from build123d import *

# Parameters (mm, degrees)
SKETCH1_W           = 200
SKETCH1_H           = 200
BOSS_EXTRUDE1_DEPTH = 30
SKETCH3_R           = 75
BOSS_EXTRUDE2_DEPTH = 30
SKETCH4_R           = 15
CUT_EXTRUDE1_DEPTH  = 30


with BuildPart() as part:
    # Sketch1 → Boss-Extrude1 (new body)
    with BuildSketch(Plane(origin=(0, 0, 0), x_dir=(1, 0, 0), z_dir=(0, 1, 0))):
        Rectangle(SKETCH1_W, SKETCH1_H)
    extrude(amount=BOSS_EXTRUDE1_DEPTH)

    # Sketch3 → Boss-Extrude2 (add)
    with BuildSketch(Plane(origin=(0, 30, 0), x_dir=(1, 0, 0), z_dir=(0, 1, 0))):
        Circle(SKETCH3_R)
    extrude(amount=BOSS_EXTRUDE2_DEPTH)

    # Sketch4 → Cut-Extrude1 (cut)
    with BuildSketch(Plane(origin=(0, 30, 0), x_dir=(1, 0, 0), z_dir=(0, 1, 0))):
        with Locations((-75, 75)):
            Circle(SKETCH4_R)
        with Locations((-75, -75)):
            Circle(SKETCH4_R)
        with Locations((75, 75)):
            Circle(SKETCH4_R)
        with Locations((75, -75)):
            Circle(SKETCH4_R)
    extrude(amount=-CUT_EXTRUDE1_DEPTH, mode=Mode.SUBTRACT)


solid = part.part
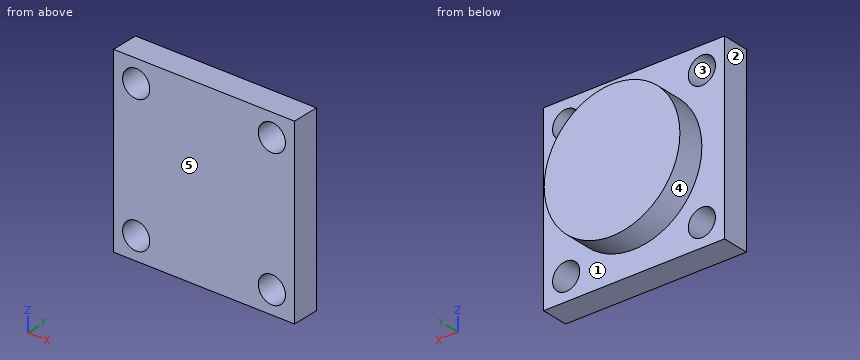
Read the model definition and answer for the solid it produces. Units are mm, in the model's axes. Face numbers are marked on the shaded views. A direction names the side the tool comes from. Give positions to 0.01 mm unless a question says otherwise; leave off trailing zeros. Write each loop counter-clockwise with the first axis right and the second up, starting at its lowest first coordinate (ties: lowest second). Pieces come first, ordered by that corner, then holes. Notation, with made-up numbers: (15, 84) - (73, 84) arc R4 ccw to (73, 88) - close; hole circle Ø7 at (1, -8.5). An arc over 180 degrees is marked (long way). Use CSV: the item, a comma, the result in double quotes. Start each with the question number.
Item 1: The part is cut by section D-D, the plane x = 80. Give the vertices of the cut face in (y, z).
Item 2: Flat-ended cylindrical pins translate along their axes: P1, Ø4, axis at x = 27, y = 35.5, coming from the -Z side; P2, Ø18, axis at x = -75, z = 75, coming from the -Y side; P3, Ø6, axis at x = -47, y = 42, coming from the -Z side. Find the tip coordinate at first contact, or state that the pin passes through.
Item 3: The part is cut by section C-C, the plane x = 0. Give the vertices of the cut face in (y, z).
Item 4: The part is cut by section A-A, the plane y = 21. Give the vertices of the cut face in (x, z), and give its area (3 significant figures).
Item 5: Consider line 1 (X direction, y = 7.25, z = 75); line 2 (X direction, y = 22, z = -64). Determine where each line is inside the solid, lowest interval first.
Item 6: For the marked faces 4 and 5, determine the directions among +Z, -Z, +X, -X, +Y, -Y from which every point of the face is accessible in a straight line to the end or side of a thin tool.
Item 7: The mould has two halves that part along X. Classify the marked faces 1, 2 and 3: pulls with the +X half, pulls with the -X half, needs draft (parallel to the pull), parting line crosses it, or undercut.
Item 8: The part is cut by section B-B, the plane z = 0. Give the vertices of the cut face in (x, y).
Taken from the geometry:
1,outline,"(0, -100) - (30, -100) - (30, -89.14) - (0, -89.14) - close; (0, -60.86) - (30, -60.86) - (30, 60.86) - (0, 60.86) - close; (0, 89.14) - (30, 89.14) - (30, 100) - (0, 100) - close"
2,P1,"z = -70.71"
2,P2,"through"
2,P3,"z = -60.74"
3,outline,"(0, -100) - (30, -100) - (30, -75) - (60, -75) - (60, 75) - (30, 75) - (30, 100) - (0, 100) - close"
4,outline,"(-100, -100) - (100, -100) - (100, 100) - (-100, 100) - close; hole circle Ø30 at (-75, -75); hole circle Ø30 at (-75, 75); hole circle Ø30 at (75, -75); hole circle Ø30 at (75, 75)"
4,area,"37,200 mm2"
5,line 1,"-100 to -90, -60 to 60, 90 to 100"
5,line 2,"-100 to -85.2, -64.8 to 64.8, 85.2 to 100"
6,face 4,"+Y"
6,face 5,"+Z, -Z, +X, -X, -Y"
7,face 1,"needs draft"
7,face 2,"pulls with the -X half"
7,face 3,"undercut"
8,outline,"(-100, 0) - (100, 0) - (100, 30) - (75, 30) - (75, 60) - (-75, 60) - (-75, 30) - (-100, 30) - close"
